Check sheet for the modelled part. Datum: model origin and axes. Units: mm. A direction names the side the tool comes from. Give positions to 0.01 mm unless a question says otherwise; leave off trailing zeros. Order: outer loops, then holes, each group sorted by start corner. A loop starts at its lowest first (then second) coordinate and runs counter-clockwise, first axis right, second up. Notation, with made-up numbers: (6, 50.25) -> (17, 50.25) arc R26 cw to (17, 85.25) -> close; hole circle Ø7 at (46.25, 49.5). An arc over 180 degrees is marked (long way). One line per question, with ' | ' between items.
```python
from build123d import *

# Parameters (mm, degrees)
BOSS_EXTRUDE1_DEPTH = 196
CUT_EXTRUDE4_REACH  = 17
SKETCH5_R           = 2.25
CUT_EXTRUDE5_REACH  = 14
SKETCH6_R           = 2.25


with BuildPart() as part:
    # Sketch1 → Boss-Extrude1 (new body)
    with BuildSketch(Plane(origin=(0, 0, 0), x_dir=(1, 0, 0), z_dir=(0, 1, 0))):
        Polygon((0, 0), (15, 0), (15, 12), (13, 12), (13, 2), (0, 2), align=None)
    extrude(amount=BOSS_EXTRUDE1_DEPTH)

    # Sketch5 → Cut-Extrude4 (cut, up to next)
    with BuildSketch(Plane(origin=(15, 0, 0), x_dir=(0, 0, -1), z_dir=(1, 0, 0)), mode=Mode.PRIVATE) as cut_extrude4_sk1:
        with Locations((4.5, 23)):
            Circle(SKETCH5_R)
    cut_extrude4_tool1 = extrude(cut_extrude4_sk1.sketch, amount=-CUT_EXTRUDE4_REACH, mode=Mode.PRIVATE) & part.part
    add(cut_extrude4_tool1.solids().sort_by_distance((15, 23, -4.5))[0], mode=Mode.SUBTRACT)
    # Sketch5 → Cut-Extrude4 (cut, up to next)
    with BuildSketch(Plane(origin=(15, 0, 0), x_dir=(0, 0, -1), z_dir=(1, 0, 0)), mode=Mode.PRIVATE) as cut_extrude4_sk2:
        with Locations((4.5, 55.5)):
            Circle(SKETCH5_R)
    cut_extrude4_tool2 = extrude(cut_extrude4_sk2.sketch, amount=-CUT_EXTRUDE4_REACH, mode=Mode.PRIVATE) & part.part
    add(cut_extrude4_tool2.solids().sort_by_distance((15, 55.5, -4.5))[0], mode=Mode.SUBTRACT)
    # Sketch5 → Cut-Extrude4 (cut, up to next)
    with BuildSketch(Plane(origin=(15, 0, 0), x_dir=(0, 0, -1), z_dir=(1, 0, 0)), mode=Mode.PRIVATE) as cut_extrude4_sk3:
        with Locations((4.5, 88)):
            Circle(SKETCH5_R)
    cut_extrude4_tool3 = extrude(cut_extrude4_sk3.sketch, amount=-CUT_EXTRUDE4_REACH, mode=Mode.PRIVATE) & part.part
    add(cut_extrude4_tool3.solids().sort_by_distance((15, 88, -4.5))[0], mode=Mode.SUBTRACT)
    # Sketch5 → Cut-Extrude4 (cut, up to next)
    with BuildSketch(Plane(origin=(15, 0, 0), x_dir=(0, 0, -1), z_dir=(1, 0, 0)), mode=Mode.PRIVATE) as cut_extrude4_sk4:
        with Locations((4.5, 108)):
            Circle(SKETCH5_R)
    cut_extrude4_tool4 = extrude(cut_extrude4_sk4.sketch, amount=-CUT_EXTRUDE4_REACH, mode=Mode.PRIVATE) & part.part
    add(cut_extrude4_tool4.solids().sort_by_distance((15, 108, -4.5))[0], mode=Mode.SUBTRACT)
    # Sketch5 → Cut-Extrude4 (cut, up to next)
    with BuildSketch(Plane(origin=(15, 0, 0), x_dir=(0, 0, -1), z_dir=(1, 0, 0)), mode=Mode.PRIVATE) as cut_extrude4_sk5:
        with Locations((4.5, 140.5)):
            Circle(SKETCH5_R)
    cut_extrude4_tool5 = extrude(cut_extrude4_sk5.sketch, amount=-CUT_EXTRUDE4_REACH, mode=Mode.PRIVATE) & part.part
    add(cut_extrude4_tool5.solids().sort_by_distance((15, 140.5, -4.5))[0], mode=Mode.SUBTRACT)
    # Sketch5 → Cut-Extrude4 (cut, up to next)
    with BuildSketch(Plane(origin=(15, 0, 0), x_dir=(0, 0, -1), z_dir=(1, 0, 0)), mode=Mode.PRIVATE) as cut_extrude4_sk6:
        with Locations((4.5, 173)):
            Circle(SKETCH5_R)
    cut_extrude4_tool6 = extrude(cut_extrude4_sk6.sketch, amount=-CUT_EXTRUDE4_REACH, mode=Mode.PRIVATE) & part.part
    add(cut_extrude4_tool6.solids().sort_by_distance((15, 173, -4.5))[0], mode=Mode.SUBTRACT)

    # Sketch6 → Cut-Extrude5 (cut, up to next)
    with BuildSketch(Plane.XY, mode=Mode.PRIVATE) as cut_extrude5_sk1:
        with Locations((7.5, 23.833333333)):
            Circle(SKETCH6_R)
    cut_extrude5_tool1 = extrude(cut_extrude5_sk1.sketch, amount=-CUT_EXTRUDE5_REACH, mode=Mode.PRIVATE) & part.part
    add(cut_extrude5_tool1.solids().sort_by_distance((7.5, 23.833333, 0))[0], mode=Mode.SUBTRACT)
    # Sketch6 → Cut-Extrude5 (cut, up to next)
    with BuildSketch(Plane.XY, mode=Mode.PRIVATE) as cut_extrude5_sk2:
        with Locations((7.5, 57.166666667)):
            Circle(SKETCH6_R)
    cut_extrude5_tool2 = extrude(cut_extrude5_sk2.sketch, amount=-CUT_EXTRUDE5_REACH, mode=Mode.PRIVATE) & part.part
    add(cut_extrude5_tool2.solids().sort_by_distance((7.5, 57.166667, 0))[0], mode=Mode.SUBTRACT)
    # Sketch6 → Cut-Extrude5 (cut, up to next)
    with BuildSketch(Plane.XY, mode=Mode.PRIVATE) as cut_extrude5_sk3:
        with Locations((7.5, 90.5)):
            Circle(SKETCH6_R)
    cut_extrude5_tool3 = extrude(cut_extrude5_sk3.sketch, amount=-CUT_EXTRUDE5_REACH, mode=Mode.PRIVATE) & part.part
    add(cut_extrude5_tool3.solids().sort_by_distance((7.5, 90.5, 0))[0], mode=Mode.SUBTRACT)
    # Sketch6 → Cut-Extrude5 (cut, up to next)
    with BuildSketch(Plane.XY, mode=Mode.PRIVATE) as cut_extrude5_sk4:
        with Locations((7.5, 105.5)):
            Circle(SKETCH6_R)
    cut_extrude5_tool4 = extrude(cut_extrude5_sk4.sketch, amount=-CUT_EXTRUDE5_REACH, mode=Mode.PRIVATE) & part.part
    add(cut_extrude5_tool4.solids().sort_by_distance((7.5, 105.5, 0))[0], mode=Mode.SUBTRACT)
    # Sketch6 → Cut-Extrude5 (cut, up to next)
    with BuildSketch(Plane.XY, mode=Mode.PRIVATE) as cut_extrude5_sk5:
        with Locations((7.5, 138.833333333)):
            Circle(SKETCH6_R)
    cut_extrude5_tool5 = extrude(cut_extrude5_sk5.sketch, amount=-CUT_EXTRUDE5_REACH, mode=Mode.PRIVATE) & part.part
    add(cut_extrude5_tool5.solids().sort_by_distance((7.5, 138.833333, 0))[0], mode=Mode.SUBTRACT)
    # Sketch6 → Cut-Extrude5 (cut, up to next)
    with BuildSketch(Plane.XY, mode=Mode.PRIVATE) as cut_extrude5_sk6:
        with Locations((7.5, 172.166666667)):
            Circle(SKETCH6_R)
    cut_extrude5_tool6 = extrude(cut_extrude5_sk6.sketch, amount=-CUT_EXTRUDE5_REACH, mode=Mode.PRIVATE) & part.part
    add(cut_extrude5_tool6.solids().sort_by_distance((7.5, 172.166667, 0))[0], mode=Mode.SUBTRACT)


solid = part.part
```
Q1. Mould release check, pull along Y, two halves, no side actions. Record for faces 1 (the face through (14.014, 85.804, -4.012)), 2 (the face through (13, 97, -7)), 3 (the face through (9.7, 0, -1.6)): pulls with the +Y half, pulls with the -Y half, needs draft (parallel to the pull), parting line crosses it, or undercut.
Result sheet:
face 1: undercut | face 2: needs draft | face 3: pulls with the -Y half
Q2. Section check B-B (z = -4.75). Enter the section's corners in (x, y).
Result sheet:
outline: (13, 0) -> (15, 0) -> (15, 20.76) -> (13, 20.76) -> close; (13, 25.24) -> (15, 25.24) -> (15, 53.26) -> (13, 53.26) -> close; (13, 57.74) -> (15, 57.74) -> (15, 85.76) -> (13, 85.76) -> close; (13, 90.24) -> (15, 90.24) -> (15, 105.76) -> (13, 105.76) -> close; (13, 110.24) -> (15, 110.24) -> (15, 138.26) -> (13, 138.26) -> close; (13, 142.74) -> (15, 142.74) -> (15, 170.76) -> (13, 170.76) -> close; (13, 175.24) -> (15, 175.24) -> (15, 196) -> (13, 196) -> close
Q3. Section check C-C (y = 61). Enter the section's corners in (x, z).
Result sheet:
outline: (0, -2) -> (13, -2) -> (13, -12) -> (15, -12) -> (15, 0) -> (0, 0) -> close
Q4. Section check A-A (x = 7.5). Enter the section's corners in (y, z), and give its area (3 significant figures).
Result sheet:
outline: (0, -2) -> (21.58, -2) -> (21.58, 0) -> (0, 0) -> close; (26.08, -2) -> (54.92, -2) -> (54.92, 0) -> (26.08, 0) -> close; (59.42, -2) -> (88.25, -2) -> (88.25, 0) -> (59.42, 0) -> close; (92.75, -2) -> (103.25, -2) -> (103.25, 0) -> (92.75, 0) -> close; (107.75, -2) -> (136.58, -2) -> (136.58, 0) -> (107.75, 0) -> close; (141.08, -2) -> (169.92, -2) -> (169.92, 0) -> (141.08, 0) -> close; (174.42, -2) -> (196, -2) -> (196, 0) -> (174.42, 0) -> close | area: 338 mm2
Q5. Depth check by flat-ended pin: pin 1 Ø6 at (x, y) = (7.5, 90.5) entering from -Z; pin 2 Ø5 at (y, z) = (58.5, -5) entering from -X. Enter the tip coordinate at first touch or a pass-through.
Result sheet:
pin 1: stops at z = -2 | pin 2: stops at x = 13
Q6. Thickness scan on line 1 (X direction, y = 80, z = -10); line 2 (Z direction, x = 9.5, y = 175.5). Record the ranges inside material, lowest first.
Result sheet:
line 1: x = 13 to 15 | line 2: z = -2 to 0
Q7. Access from +Z, -Z, +X, -X, +Y, -Y to the whole of each face (thin tool, end or side, straight path). Record for faces 4 (the face through (7.207, 26.064, -0.986)), 5 (the face through (7, 97, -2)).
Result sheet:
face 4: +Z, -Z | face 5: -Z, -X, +Y, -Y
